```python
from build123d import *

# Parameters (mm, degrees)
F3_W     = 12
F3_H     = 6
F0_DEPTH = 6.0000000522
F1_R     = 1.5
F4_DEPTH = 2
F5_SIZE  = 0.3
F2_T     = 1


# Not quite as in the source:
# - a shell that OpenCascade refuses in one call is made with other operations: the cavity is built on its own and cut out


with BuildPart() as f0:
    # F3 (on Top) → F0 (new body)
    with BuildSketch(Plane.XY):
        Rectangle(F3_W, F3_H)
    extrude(amount=-F0_DEPTH)

    # F1 (on Top) → F4 (join)
    with BuildSketch(Plane.XY):
        with Locations((3, 0)):
            Circle(F1_R)
        with Locations((-3, 0)):
            Circle(F1_R)
    extrude(amount=F4_DEPTH)

    # F5
    f5_edges = [f0.edges().sort_by_distance(p)[0] for p in [
        (-4.5, 0, 2),
        (1.5, 0, 2),
    ]]
    chamfer(f5_edges, length=F5_SIZE)

    # F2: shell of thickness 1, made by hand


with BuildPart() as f2_core1:
    # F2_t2: copy of F0
    add(f0.part)

    # the walls: a layer under each face that stays
    f2_faces = [f2_core1.faces().sort_by_distance(p)[0] for p in [
        (-4.5, 0, 0.85),
        (-4.35, 0, 1.85),
        (0, 0, 0),
        (-3, 0, 2),
        (0, 3, -3.0000000261),
        (6, 0, -3.0000000261),
        (-6, 0, -3.0000000261),
        (0, -3, -3.0000000261),
        (1.5, 0, 0.85),
        (1.65, 0, 1.85),
        (3, 0, 2),
    ]]
    thicken(f2_faces, amount=-F2_T, mode=Mode.SUBTRACT)

    # F2_s3 → F2_t4 (revolve, cut)
    with BuildSketch(Plane.XZ):
        Polygon((-1.49, 0.01), (-2.5, 0), (-2.5, -1), (-1.5, -1), align=None)
    revolve(axis=Axis((-3, 0, 0), (0, 0, 1)), mode=Mode.SUBTRACT)

    # F2_s5 → F2_t6 (revolve, cut)
    with BuildSketch(Plane.XZ):
        Polygon((4.51, 0.01), (4.5, -1), (3.5, -1), (3.5, 0), align=None)
    revolve(axis=Axis((3, 0, 0), (0, 0, 1)), mode=Mode.SUBTRACT)


with BuildPart() as f0_1:
    add(f0.part)

    # what is left inside the walls is the cavity
    f2_cavity = [f2_core1.part.solids().sort_by_distance(p)[0] for p in [
        (0, 1.99, -4.333333),
    ]]
    add(f2_cavity, mode=Mode.SUBTRACT)


solid = f0_1.part
```
CAD build for the part. Positions are in the model's coordinates, mm. A direction names the side the tool comes from. Coordinates: 2 decimals unless noted, no trailing zeros. Write each loop counter-clockwise with the first axis right and the second up, starting at its lowest first coordinate (ties: lowest second). Pieces come first, ordered by that corner, then holes.
(1) Two-plate mould, pull along Y, no slides. Class faces 1 (the face through (0, -3, -3)), 2 (the face through (-3, 0, 2)), 3 (the face through (5, 0, -3)): +Y half, -Y half, draft (parallel to the pull), parting line (faces both ways), or undercut.
(2) Cut at C-C, the plane z = 0.5. List the corners of the cut face in (x, y), and give its area (3 significant figures).
(3) 3-axis set-ups, long thin cutter, end or side, ignore diameter. For faces 4 (the face through (-1.57, 0.45, 0.84)), 5 (the face through (3, 0, 2)), 6 (the face through (0, 2, -3)): which of +Z, -Z, +X, -X, +Y, -Y reach the whole face in a straight line?
(4) Drill centre lines: probe 1 along X at (y, z) = (0, -0.05); probe 2 along Y at (x, z) = (3, -0.25); probe 3 along X at (y, z) = (1.45, -2.5). Where is each one in solid material? Low to high.
(5) Cut at A-A, the plane z = -4. List the corners of the cut face in (x, y), and give its area (3 significant figures).
(6) Cut at D-D, the plane x = 3. List the corners of the cut face in (y, z), and give its area (3 significant figures).
(7) Cut at B-B, the plane y = -1.85. List the corners of the cut face in (x, z).
(8) Flat gauge pins, fed straight in: pin 1 (0.5 mm diameter, centred on x = -3, y = 0, fed in from -Z); pin 2 (1.8 mm diameter, centred on x = 0, y = 1, fed in from +Z). Where does each tip first touch, or does it go through?
Geometry says:
1. face 1: -Y half
1. face 2: draft
1. face 3: undercut
2. outline: circle Ø3 at (-3, 0); circle Ø3 at (3, 0); hole circle Ø1 at (-3, 0); hole circle Ø1 at (3, 0)
2. area: 12.6 mm2
3. face 4: +Z
3. face 5: +Z, +X, -X, +Y, -Y
3. face 6: -Z
4. probe 1: x = -6 to -3.5, -2.5 to 2.5, 3.5 to 6
4. probe 2: y = -3 to -0.5, 0.5 to 3
4. probe 3: x = -6 to -5, 5 to 6
5. outline: (-6, -3) - (6, -3) - (6, 3) - (-6, 3) - close; hole (-5, -2) - (5, -2) - (5, 2) - (-5, 2) - close
5. area: 32.0 mm2
6. outline: (-3, -6) - (-2, -6) - (-2, -1) - (-0.5, -1) - (-0.5, 1) - (0.5, 1) - (0.5, -1) - (2, -1) - (2, -6) - (3, -6) - (3, 0) - (1.5, 0) - (1.5, 1.7) - (1.2, 2) - (-1.2, 2) - (-1.5, 1.7) - (-1.5, 0) - (-3, 0) - close
6. area: 19.9 mm2
7. outline: (-6, -6) - (-5, -6) - (-5, -1) - (5, -1) - (5, -6) - (6, -6) - (6, 0) - (-6, 0) - close
8. pin 1: stops at z = 1
8. pin 2: stops at z = 0
